```python
from build123d import *

# Parameters (mm, degrees)
SKETCH1_W           = 1.5
SKETCH1_H           = 8
BOSS_EXTRUDE1_DEPTH = 0.5
SKETCH2_W           = 0.05
SKETCH2_H           = 0.5
BOSS_EXTRUDE2_DEPTH = 8
SKETCH3_W           = 8
SKETCH3_H           = 0.3
CUT_EXTRUDE1_DEPTH  = 14.095800854


with BuildPart() as part:
    # Sketch1 → Boss-Extrude1 (new body)
    with BuildSketch(Plane(origin=(0, 0, 0), x_dir=(0, 1, 0), z_dir=(0, 0, 1))):
        with Locations((1.25, -5)):
            Rectangle(SKETCH1_W, SKETCH1_H)
    extrude(amount=BOSS_EXTRUDE1_DEPTH)

    # Sketch2 → Boss-Extrude2 (add)
    with BuildSketch(Plane(origin=(0, 2, 0), x_dir=(-1, 0, 0), z_dir=(0, 1, 0))):
        with Locations((-8.75, 0.25)):
            Rectangle(SKETCH2_W, SKETCH2_H)
        with Locations((-8.25, 0.25)):
            Rectangle(SKETCH2_W, SKETCH2_H)
        with Locations((-7.75, 0.25)):
            Rectangle(SKETCH2_W, SKETCH2_H)
        with Locations((-7.25, 0.25)):
            Rectangle(SKETCH2_W, SKETCH2_H)
        with Locations((-6.75, 0.25)):
            Rectangle(SKETCH2_W, SKETCH2_H)
        with Locations((-6.25, 0.25)):
            Rectangle(SKETCH2_W, SKETCH2_H)
        with Locations((-5.75, 0.25)):
            Rectangle(SKETCH2_W, SKETCH2_H)
        with Locations((-5.25, 0.25)):
            Rectangle(SKETCH2_W, SKETCH2_H)
        with Locations((-4.75, 0.25)):
            Rectangle(SKETCH2_W, SKETCH2_H)
        with Locations((-4.25, 0.25)):
            Rectangle(SKETCH2_W, SKETCH2_H)
        with Locations((-3.75, 0.25)):
            Rectangle(SKETCH2_W, SKETCH2_H)
        with Locations((-3.25, 0.25)):
            Rectangle(SKETCH2_W, SKETCH2_H)
        with Locations((-2.75, 0.25)):
            Rectangle(SKETCH2_W, SKETCH2_H)
        with Locations((-2.25, 0.25)):
            Rectangle(SKETCH2_W, SKETCH2_H)
        with Locations((-1.75, 0.25)):
            Rectangle(SKETCH2_W, SKETCH2_H)
        with Locations((-1.25, 0.25)):
            Rectangle(SKETCH2_W, SKETCH2_H)
    extrude(amount=BOSS_EXTRUDE2_DEPTH)

    # Sketch3 → Cut-Extrude1 (cut, through all)
    with BuildSketch(Plane.XZ.offset(-0.5)):
        with Locations((5, 0.15)):
            Rectangle(SKETCH3_W, SKETCH3_H)
    extrude(amount=-CUT_EXTRUDE1_DEPTH, mode=Mode.SUBTRACT)


solid = part.part
```
The listing builds one solid part. Answer for the finished solid, in the listing's coordinates (mm). Give positions to 0.01 mm unless a question says otherwise; leave off trailing zeros. Loops run counter-clockwise (first coordinate to the right, second up) from the corner with the lowest first, then second, coordinate; pieces in that order, holes last. Notation, with made-up numbers: (62, 66.5) - (91, 66.5) arc R11 ccw to (91, 85.5) - close; hole circle Ø1 at (81.25, 4.25). An arc over 180 degrees is marked (long way). Answer as CSV lines item,"result". Start each with the question number.
Item 1: A cutting plane is placed at B-B on x = 7. Determine the outline of the cut face in (y, z).
Item 2: A cutting plane is placed at A-A on y = 4. Count the separate pieces of the cut face and the enclosed holes in it, then the cut area to 3 significant figures.
Item 3: Find the intervals of material crossed by line 1 (Y direction, x = 3.5, z = 0.4), in increasing order. Write a range as from..to.
Found:
1,outline,"(0.5, 0.3) - (2, 0.3) - (2, 0.5) - (0.5, 0.5) - close"
2,separate pieces,"16"
2,enclosed holes,"0"
2,area,"0.160 mm^2"
3,line 1,"y = 0.5..2"
